from build123d import *

# Parameters (mm, degrees)
BASPROSKE_W             = 5.5
BASPROSKE_H             = 5.5
TOOTHCUT_DEPTH          = 10.526279442
TEETHCUTS_COUNT         = 20
TEETHCUTS_ANGLE         = 342
BORSKE_R                = 0.5
BORE_DEPTH              = 50.0008636
CUT_EXTRUDE1_DEPTH      = 10.476593643
CUT_EXTRUDE1_DEPTH_BACK = 10.476593643
SKETCH3_R               = 3.65
SKETCH3_R_2             = 1.35
BOSS_EXTRUDE1_DEPTH     = 2.5


with BuildPart() as part:
    # BasProSke → Base-Revolve (revolve)
    with BuildSketch(Plane(origin=(0, 0, 0), x_dir=(1, 0, 0), z_dir=(0, 1, 0)), mode=Mode.PRIVATE) as base_revolve_sk:
        with Locations((2.75, 2.75)):
            Rectangle(BASPROSKE_W, BASPROSKE_H)
    revolve(base_revolve_sk.sketch.rotate(Axis((-10, 0, 0), (1, 0, 0)), 180), axis=Axis((-10, 0, 0), (1, 0, 0)))

    # TooCutSke → ToothCut (cut, through all)
    with BuildSketch(Plane(origin=(0, 0, 0), x_dir=(0, 0, -1), z_dir=(1, 0, 0))):
        with BuildLine():
            ThreePointArc((0.29465164, 4.364064208), (0, 4.374), (-0.29465164, 4.364064208))
            ThreePointArc((-0.29465164, 4.364064208), (-0.414807829, 4.95335164), (-0.704719584, 5.480275127))
            ThreePointArc((-0.704719584, 5.480275127), (0, 5.5254), (0.704719584, 5.480275127))
            ThreePointArc((0.704719584, 5.480275127), (0.414807829, 4.95335164), (0.29465164, 4.364064208))
        make_face()
    toothcut = extrude(amount=TOOTHCUT_DEPTH, mode=Mode.SUBTRACT)

    # TeethCuts: ToothCut ×20 about axis
    teethcuts_axis = Axis((-10, 0, 0), (1, 0, 0))
    for i in range(1, TEETHCUTS_COUNT):
        add(toothcut.rotate(teethcuts_axis, i * TEETHCUTS_ANGLE / (TEETHCUTS_COUNT - 1)), mode=Mode.SUBTRACT)

    # BorSke → Bore (cut, symmetric)
    with BuildSketch(Plane(origin=(0, 0, 0), x_dir=(0, 0, -1), z_dir=(1, 0, 0))):
        with Locations(Location((0, 0, 0), (0, 0, 180))):
            Circle(BORSKE_R)
    extrude(amount=BORE_DEPTH, both=True, mode=Mode.SUBTRACT)

    # Sketch2 → Cut-Extrude1 (cut, two sides: drawn at the far end of the back side and taken through both)
    with BuildSketch(Plane.ZY.offset(-CUT_EXTRUDE1_DEPTH_BACK)):
        with BuildLine():
            Line((-1.777198988, 2.623027169), (-1.87625046, 1.9300706))
            Line((-1.87625046, 1.9300706), (-2.371433872, 1.873523785))
            Line((-2.371433872, 1.873523785), (-2.311857805, 1.378695687))
            Line((-2.311857805, 1.378695687), (-2.963084724, 1.121978916))
            ThreePointArc((-2.963084724, 1.121978916), (-3.135124987, 0.457929127), (-3.160207657, -0.227585887))
            Line((-3.160207657, -0.227585887), (-2.6096154, -0.659845262))
            Line((-2.6096154, -0.659845262), (-2.808236128, -1.116960084))
            Line((-2.808236128, -1.116960084), (-2.349914391, -1.312779746))
            Line((-2.349914391, -1.312779746), (-2.453204606, -2.005117186))
            ThreePointArc((-2.453204606, -2.005117186), (-1.964140751, -2.48613332), (-1.383008669, -2.850613056))
            Line((-1.383008669, -2.850613056), (-0.733364941, -2.589915862))
            Line((-0.733364941, -2.589915862), (-0.436802256, -2.990483869))
            Line((-0.436802256, -2.990483869), (-0.038056586, -2.691475433))
            Line((-0.038056586, -2.691475433), (0.509880118, -3.127096103))
            ThreePointArc((0.509880118, -3.127096103), (1.170984237, -2.944062446), (1.777198988, -2.623027169))
            Line((1.777198988, -2.623027169), (1.87625046, -1.9300706))
            Line((1.87625046, -1.9300706), (2.371433872, -1.873523785))
            Line((2.371433872, -1.873523785), (2.311857805, -1.378695687))
            Line((2.311857805, -1.378695687), (2.963084724, -1.121978916))
            ThreePointArc((2.963084724, -1.121978916), (3.135124987, -0.457929127), (3.160207657, 0.227585887))
            Line((3.160207657, 0.227585887), (2.6096154, 0.659845262))
            Line((2.6096154, 0.659845262), (2.808236128, 1.116960084))
            Line((2.808236128, 1.116960084), (2.349914391, 1.312779746))
            Line((2.349914391, 1.312779746), (2.453204606, 2.005117186))
            ThreePointArc((2.453204606, 2.005117186), (1.964140751, 2.48613332), (1.383008669, 2.850613056))
            Line((1.383008669, 2.850613056), (0.733364941, 2.589915862))
            Line((0.733364941, 2.589915862), (0.436802256, 2.990483869))
            Line((0.436802256, 2.990483869), (0.038056586, 2.691475433))
            Line((0.038056586, 2.691475433), (-0.509880118, 3.127096103))
            ThreePointArc((-0.509880118, 3.127096103), (-1.170984237, 2.944062446), (-1.777198988, 2.623027169))
        make_face()
    extrude(amount=CUT_EXTRUDE1_DEPTH + CUT_EXTRUDE1_DEPTH_BACK, mode=Mode.SUBTRACT)

    # Sketch3 → Boss-Extrude1 (add)
    with BuildSketch(Plane.ZY):
        Circle(SKETCH3_R)
        Circle(SKETCH3_R_2, mode=Mode.SUBTRACT)
    extrude(amount=-BOSS_EXTRUDE1_DEPTH)


solid = part.part
Source: CAD feature listing. Evaluate the final solid. Frame: model axes, mm. A direction names the side the tool comes from. Round coordinates to 2 decimals unless told otherwise and drop trailing zeros. Loops run counter-clockwise (first coordinate to the right, second up) from the corner with the lowest first, then second, coordinate; pieces in that order, holes last. Notation, with made-up numbers: M 45,1.25 L 59,1.25 A35 ccw 59,40.25 Z; hole C 81.5,72.25 d7. An arc over 180 degrees is marked long. Answer as CSV lines item,"result".
Q1. Contact query for flat-ended pins moving along their axis: pin 1 (2 mm diameter, centred on x = 1, y = -1, fed in from +Z); pin 2 (1.5 mm diameter, centred on x = 2, y = -2, fed in from -Z). Output: stop coordinate, or through.
Verdict:
pin 1,"stops at z = 5.46"
pin 2,"stops at z = -4.98"
Q2. Cut plane B-B (y = 3.5). Return the cut outline in (x, z), plus the area to 3 significant figures.
Verdict:
outline,"M 0,-3.91 L 5.5,-3.91 L 5.5,-2.93 L 0,-2.93 Z; M 0,-2.62 L 5.5,-2.62 L 5.5,2.62 L 0,2.62 Z; M 0,2.93 L 5.5,2.93 L 5.5,3.91 L 0,3.91 Z"
area,"39.6 mm^2"
Q3. Cut plane A-A (y = 0). Return the cut outline in (x, z).
Verdict:
outline,"M 0,-4.37 L 5.5,-4.37 L 5.5,-3.17 L 2.5,-3.17 L 2.5,-1.35 L 0,-1.35 Z; M 0,1.35 L 2.5,1.35 L 2.5,3.17 L 5.5,3.17 L 5.5,4.37 L 0,4.37 Z"
Q4. Line query: line 1 along Y through (x, z) = (0.75, 0); line 2 along Y through (x, z) = (3.1, 2.75); line 3 along Y through (x, z) = (2.3, -3.5). Output: solid intervals per line, ascending.
Verdict:
line 1,"y = -4.37 to -1.35, 1.35 to 4.37"
line 2,"y = -3.4 to -1.21, 0.55 to 0.98, 1.14 to 3.4"
line 3,"y = -3.91 to -2.93, -2.62 to 2.62, 2.93 to 3.91"
Q5. Pull-direction query (Z, two-part tool) for faces 6 (the face through (2.712, 1.921, 4.578)), 7 (the face through (2.71, -3.24, -3.76)), 8 (the face through (0, 1.1, -1.1)), 9 (the face through (2.712, 1.137, 4.816)); classes: +Z half, -Z half, draft (parallel to the pull), parting line (faces both ways), or undercut.
Verdict:
face 6,"+Z half"
face 7,"-Z half"
face 8,"draft"
face 9,"undercut"
Q6. Reachability of faces 1 (the face through (2.71, -3.75, -3.23)), 2 (the face through (2.71, 1.91, -4.56)), 3 (the face through (2.712, -4.833, -1.136)), 4 (the face through (2.71, 3.76, -3.24)), 5 (the face through (2.712, -0.407, 4.932)) from +Z, -Z, +X, -X, +Y, -Y: full face, straight path, thin tool, end or side. Return the list, or none.
Verdict:
face 1,"+X, -X, -Y"
face 2,"-Z, +X, -X"
face 3,"+X, -X"
face 4,"+X, -X, +Y"
face 5,"+Z, +X, -X"
